Model file for the job. Use its own axes, mm. A direction names the side the tool comes from. Round coordinates to 2 decimals unless told otherwise and drop trailing zeros. Order: outer loops, then holes, each group sorted by start corner. A loop starts at its lowest first (then second) coordinate and runs counter-clockwise, first axis right, second up. Notation, with made-up numbers: M -14.5,-19 L -3.5,-19 A27 cw -3.5,0 Z; hole C 19,0 d2. An arc over 180 degrees is marked long. Return JSON: item names as keys, results as strings. Group by question number.
Item 1: Pull direction Y, two halves, no side cores. Call faces 4 (the face through (-13, -0.685, 1)), 5 (the face through (-25, 21.315, 1)), 6 (the face through (3, 28, 1)), 7 (the face through (-20.952, 11.229, 1.479)): pulls with the +Y half, pulls with the -Y half, needs draft (parallel to the pull), parting line crosses it, or undercut.
Item 2: Probe line 1 along Y through (x, z) = (-11.5, 2) (3 decimals); line 2 along Y through (x, z) = (-16, 1.65) (3 decimals); line 3 along X through (y, z) = (17, 2.3). List the from-to ranges inside material, lowest first.
Item 3: Slice it at A-A on x = -19. Write the cut outline in (y, z) (3 decimals), then the cut area to 3 significant figures.
Item 4: Slice it at C-C on z = 2. Write the cut outline in (x, y) (1 decimal).
Item 5: Slice it at D-D on y = 9.17. Write the cut outline in (x, z).
Item 6: Which spindle directions (+Z, -Z, +X, -X, +Y, -Y) get a long thin tool onto all of the face, cutting with end or side? Do faces 1 (the face through (2, 18.315, 1)), 2 (the face through (0, 48, 1)), 3 (the face through (-25, 35.315, 1)). Say none if no direction does.
Item 7: Pin check, flat tips, straight feed: pin 1 Ø1.5 at (y, z) = (10, 1.5) entering from +X; pin 2 Ø0.9 at (x, z) = (2, 2) entering from +Y (3 decimals); pin 3 Ø0.9 at (x, z) = (2, 1) entering from -Y (3 decimals). Stop position of each tip, or through.
Item 8: Slice it at B-B on y = 23.5. Write the cut outline in (x, z), then the cut area to 3 significant figures.
Autodesk Inventor part; units mm, degrees
ref_plane "YZ Plane" through (0, 0, 0) normal (1, 0, 0) x (0, 1, 0)
ref_plane "XZ Plane" through (0, 0, 0) normal (0, 1, 0) x (-1, 0, 0)
ref_plane "XY Plane" through (0, 0, 0) normal (0, 0, 1) x (1, 0, 0)
sketch "Sketch1" plane through (0, 0, 0) normal (0, 0, 1) x (1, 0, 0)
  circle A0 centre (-14.6869, 39.4735) radius 8.5
  circle A1 centre (-22.3409, 47.1275) radius 1.6
  circle A2 centre (-7.0512, 9.17) radius 1.6
  circle A3 centre (-8.1473, 28.508) radius 2.5
  circle A4 centre (-14.6869, 16.9735) radius 8.5
  line L0 (0, 28.315) -> (0, -0.685)
  line L1 (0, -0.685) -> (-27.2, -0.685)
  line L2 (-27.2, -0.685) -> (0, -0.685)
  line L3 (0, -0.685) -> (0, 57.315)
  line L4 (0, 57.315) -> (-27.2, 57.315)
  line L5 (-27.2, 57.315) -> (-27.2, -0.685)
  line L6 (0, 28.315) -> (0, 38.315)
  line L7 (0, 38.315) -> (3, 38.315)
  line L8 (3, 38.315) -> (3, 18.315)
  line L9 (3, 18.315) -> (0, 18.315)
  line L10 (-14.6869, 39.4735) -> (-14.6869, 28.315)
  line L11 (-14.6869, 28.315) -> (-22.6869, 28.315)
  line L12 (-22.6869, 28.315) -> (-22.6869, 21.315)
  line L13 (-22.6869, 21.315) -> (-22.6869, 35.315)
  line L14 (-22.6869, 35.315) -> (-27.2, 35.315)
  line L15 (-22.6869, 21.315) -> (-27.2, 21.315)
  point P0 (0, 0)
  point P1 (-5.6598, 20.3223)
  dimension "d1" = 29
  dimension "d2" = 58
  dimension "d3" = 10
  dimension "d4" = 3
  dimension "d5" = 20
  dimension "d10" = 8
  dimension "d11" = 7
  dimension "d12" = 14
extrude "Extrusion2" add sketch "Sketch1" along normal blind 3 contours L13 L14 L5 L4 L3 L0 L1 L15 L12 | L0 L3 L7 L8 L9
sketch "Sketch2" plane through (0, 0, 3) normal (0, 0, 1) x (1, 0, 0)
  circle A0 centre (-14.6869, 16.9735) radius 8.5
  circle A1 centre (-14.6869, 39.4735) radius 8.5
  circle A2 centre (-8.1473, 28.508) radius 2.5
  circle A3 centre (-7.0512, 9.17) radius 1.6
  circle A4 centre (-22.3409, 47.1275) radius 1.6
  line L0 (0, 18.315) -> (3, 18.315)
  line L1 (3, 18.315) -> (3, 38.315)
  line L2 (3, 38.315) -> (0, 38.315)
  line L3 (0, 38.315) -> (0, 57.315)
  line L4 (0, 57.315) -> (-27.2, 57.315)
  line L5 (-27.2, 57.315) -> (-27.2, 35.315)
  line L6 (-27.2, 35.315) -> (-22.6869, 35.315)
  line L7 (-22.6869, 35.315) -> (-22.6869, 21.315)
  line L8 (-22.6869, 21.315) -> (-27.2, 21.315)
  line L9 (-27.2, 21.315) -> (-27.2, -0.685)
  line L10 (-27.2, -0.685) -> (0, -0.685)
  line L11 (0, -0.685) -> (0, 18.315)
  line L12 (-40, 69) -> (-28.75, 69)
  point P0 (0, 0)
  dimension "d15" = 17
  dimension "d16" = 3.2
  dimension "d17" = 5
  dimension "d18" = 22.5
  dimension "d19" = 7.654
  dimension "d20" = 7.654
  dimension "d21" = 7.6357
  dimension "d22" = 7.8035
  dimension "d23" = 6.5396
  dimension "d24" = 11.5345
  dimension "d25" = 10.9655
  dimension "d26" = 11.25
equation "\"d26\" = 0.5 * d24 + 0.5 * d25"
properties part number "srf"
Output values:
{
 "1": {"face 4": "pulls with the -Y half", "face 5": "undercut", "face 6": "needs draft", "face 7": "undercut"},
 "2": {"line 1": "-0.685 to 9.094, 24.853 to 31.594, 47.353 to 57.315", "line 2": "-0.685 to 8.576, 25.371 to 31.076, 47.871 to 57.315", "line 3": "-27.2 to -23.19, -6.19 to 0"},
 "3": {"outline": "M -0.685,0 L 9.649,0 L 9.649,3 L -0.685,3 Z; M 24.298,0 L 32.149,0 L 32.149,3 L 24.298,3 Z; M 46.798,0 L 57.315,0 L 57.315,3 L 46.798,3 Z", "area": "86.1 mm²"},
 "4": {"outline": "M -27.2,-0.7 L 0,-0.7 L 0,18.3 L 3,18.3 L 3,38.3 L 0,38.3 L 0,57.3 L -27.2,57.3 L -27.2,35.3 L -22.7,35.3 L -22.7,21.3 L -27.2,21.3 Z; hole C -22.3,47.1 d3.2; hole C -14.7,17 d17; hole C -14.7,39.5 d17; hole C -8.1,28.5 d5; hole C -7.1,9.2 d3.2"},
 "5": {"outline": "M -27.2,0 L -18.06,0 L -18.06,3 L -27.2,3 Z; M -11.32,0 L -8.65,0 L -8.65,3 L -11.32,3 Z; M -5.45,0 L 0,0 L 0,3 L -5.45,3 Z"},
 "6": {"face 1": "+Z, -Z, +X, -Y", "face 2": "+Z, -Z, +X, +Y", "face 3": "+Z, -Z, -X"},
 "7": {"pin 1": "x = 0", "pin 2": "y = 38.315", "pin 3": "y = 18.315"},
 "8": {"outline": "M -22.69,0 L -20.13,0 L -20.13,3 L -22.69,3 Z; M -9.24,0 L 3,0 L 3,3 L -9.24,3 Z", "area": "44.4 mm²"}
}
